Build history of the part. All positions in model axes, mm. Face numbers are marked on the shaded views. Give positions to 0.01 mm unless a question says otherwise; leave off trailing zeros. Loops run counter-clockwise (first coordinate to the right, second up) from the corner with the lowest first, then second, coordinate; pieces in that order, holes last. Notation, with made-up numbers: (-31, 74) -> (-9, 74) arc R19 ccw to (-9, 86) -> close; hole circle Ø7 at (60.25, -19). An arc over 180 degrees is marked (long way). Answer as a JSON object with one key per item and string values. Group by question number.
Q1. Drop flat-ended pins along their axis: pin 1 (2.5 mm diameter, centred on x = 49.5, z = 15, fed in from -Y); pin 2 (1.2 mm diameter, centred on x = 98, z = 32.5, fed in from -Y); pin 3 (2 mm diameter, centred on y = -8.5, z = 10, fed in from -X); pin 4 (2 mm diameter, centred on y = -9, z = 36, fed in from -X). Give the stop position or say it passes through.
Q2. Band-saw the part on D-D, the plane x = 80. Write the cut outline in (y, z).
Q3. Band-saw the part on A-A, the plane x = 49.5. Write the cut outline in (y, z), plus the area to 3 significant figures.
Q4. Two-plate mould, pull along X, no slides. Class the marked faces 1 and 2: pulls with the +X half, pulls with the -X half, needs draft (parallel to the pull), parting line crosses it, or undercut.
Q5. Wall check: probe 1 along Z at (x, y) = (5.5, -4); probe 2 along X at (y, z) = (-4.75, 49); probe 3 along X at (y, z) = (-4.5, 15). Give the ranges that are in metal, low to high. Write a range as from..to.
Q6. Band-saw the part on C-C, the plane x = 18. Write the cut outline in (y, z), plus the area to 3 significant figures.
from build123d import *

# Parameters (mm, degrees)
BOSS_EXTRUDE1_DEPTH                  = 60
FILLET1_R                            = 1
F_2_6_START                          = -7
F_2_6_2_6_DIAMETER_HOLE1_OUTLINE_R   = 1.3
F_2_6_2_6_DIAMETER_HOLE1_DEPTH       = 7
F_2_6_START_2                        = -8.6
F_2_6_2_6_DIAMETER_HOLE1_2_OUTLINE_R = 1.3
F_2_6_2_6_DIAMETER_HOLE1_2_DEPTH     = 1.6


# Read off the part's stored shape, not the designer's step: Ø2.6 (2.6) Diameter Hole1
with BuildPart() as part:
    # Sketch1 → Boss-Extrude1 (new body)
    with BuildSketch(Plane.XY):
        with BuildLine():
            Line((0, 0), (7.751531367, 0))
            Line((7.751531367, 0), (7.751531367, -1.25))
            ThreePointArc((7.751531367, -1.25), (15.339084008, -11.30616411), (26.74540449, -5.958898944))
            Line((26.74540449, -5.958898944), (28.74540449, -5.958898944))
            ThreePointArc((28.74540449, -5.958898944), (39.981472468, -11.346794345), (47.74540449, -1.6))
            Line((47.74540449, -1.6), (51.25459551, -1.6))
            ThreePointArc((51.25459551, -1.6), (59.018527532, -11.346794345), (70.25459551, -5.958898944))
            Line((70.25459551, -5.958898944), (72.25459551, -5.958898944))
            ThreePointArc((72.25459551, -5.958898944), (83.660915992, -11.30616411), (91.248468633, -1.25))
            Line((91.248468633, -1.25), (91.248468633, 0))
            Line((91.248468633, 0), (99, 0))
            Line((99, 0), (99, -1.6))
            Line((99, -1.6), (95.52, -1.6))
            Line((95.52, -1.6), (95.52, -7))
            Line((95.52, -7), (91.970938169, -7))
            ThreePointArc((91.970938169, -7), (83.148029778, -13.449679602), (72.75459551, -10.070537173))
            Line((72.75459551, -10.070537173), (69.75459551, -10.070537173))
            ThreePointArc((69.75459551, -10.070537173), (60.290622518, -13.561218837), (51.507801165, -8.6))
            Line((51.507801165, -8.6), (47.492198835, -8.6))
            ThreePointArc((47.492198835, -8.6), (38.709377482, -13.561218837), (29.24540449, -10.070537173))
            Line((29.24540449, -10.070537173), (26.24540449, -10.070537173))
            ThreePointArc((26.24540449, -10.070537173), (15.851970222, -13.449679602), (7.029061831, -7))
            Line((7.029061831, -7), (3.48, -7))
            Line((3.48, -7), (3.48, -1.6))
            Line((3.48, -1.6), (0, -1.6))
            Line((0, -1.6), (0, 0))
        make_face()
    extrude(amount=BOSS_EXTRUDE1_DEPTH)

    # Fillet1
    fillet1_edges = [part.edges().sort_by_distance(p)[0] for p in [
        (95.52, -1.6, 30),
        (91.970938169, -7, 30),
        (7.029061831, -7, 30),
        (3.48, -1.6, 30),
    ]]
    fillet(fillet1_edges, radius=FILLET1_R)

    # Ø2.6 (2.6) Diameter Hole1 outline → Ø2.6 (2.6) Diameter Hole1 (cut)
    with BuildSketch(Plane(origin=(0, 0, 0), x_dir=(1, 0, 0), z_dir=(0, 1, 0)).offset(F_2_6_START)):
        with Locations((93.5, -15)):
            Circle(F_2_6_2_6_DIAMETER_HOLE1_OUTLINE_R)
        with Locations((93.5, -45)):
            Circle(F_2_6_2_6_DIAMETER_HOLE1_OUTLINE_R)
        with Locations((49.5, -15)):
            Circle(F_2_6_2_6_DIAMETER_HOLE1_OUTLINE_R)
        with Locations((49.5, -45)):
            Circle(F_2_6_2_6_DIAMETER_HOLE1_OUTLINE_R)
    f_2_6_2_6_diameter_hole1 = extrude(amount=F_2_6_2_6_DIAMETER_HOLE1_DEPTH, mode=Mode.SUBTRACT)

    # 2.6 _2.6_ Diameter Hole1 2 outline → 2.6 _2.6_ Diameter Hole1 2 (cut)
    with BuildSketch(Plane(origin=(0, 0, 0), x_dir=(1, 0, 0), z_dir=(0, 1, 0)).offset(F_2_6_START_2)):
        with Locations((49.5, -15)):
            Circle(F_2_6_2_6_DIAMETER_HOLE1_2_OUTLINE_R)
        with Locations((49.5, -45)):
            Circle(F_2_6_2_6_DIAMETER_HOLE1_2_OUTLINE_R)
    f_2_6_2_6_diameter_hole1_2 = extrude(amount=F_2_6_2_6_DIAMETER_HOLE1_2_DEPTH, mode=Mode.SUBTRACT)

    # Mirror1: Ø2.6 (2.6) Diameter Hole1, 2.6 _2.6_ Diameter Hole1 2 across plane
    add(f_2_6_2_6_diameter_hole1.mirror(Plane.ZY.offset(-49.5)), mode=Mode.SUBTRACT)
    add(f_2_6_2_6_diameter_hole1_2.mirror(Plane.ZY.offset(-49.5)), mode=Mode.SUBTRACT)


solid = part.part
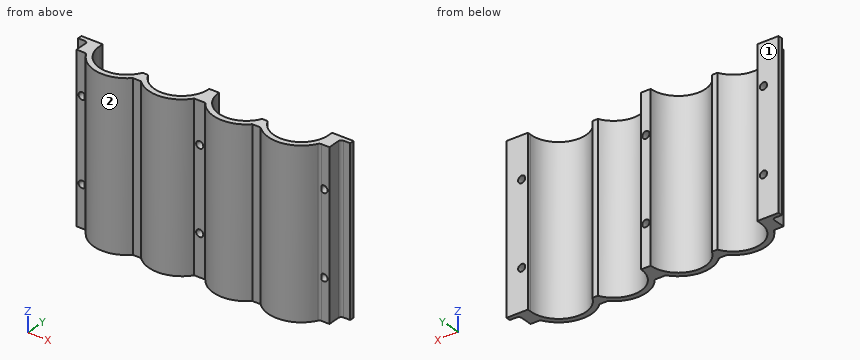
Worked answers:
{
 "1": {"pin 1": "through", "pin 2": "y = -1.6", "pin 3": "x = 7.3", "pin 4": "x = 7.59"},
 "2": {"outline": "(-13.53, 0) -> (-11.52, 0) -> (-11.52, 60) -> (-13.53, 60) -> close"},
 "3": {"outline": "(-8.6, 0) -> (-1.6, 0) -> (-1.6, 13.7) -> (-8.6, 13.7) -> close; (-8.6, 16.3) -> (-1.6, 16.3) -> (-1.6, 43.7) -> (-8.6, 43.7) -> close; (-8.6, 46.3) -> (-1.6, 46.3) -> (-1.6, 60) -> (-8.6, 60) -> close", "area": "384 mm2"},
 "4": {"face 1": "needs draft", "face 2": "undercut"},
 "5": {"probe 1": "0..13.7, 16.3..43.7, 46.3..60", "probe 2": "3.48..8.25, 47.24..51.76, 90.75..95.52", "probe 3": "3.48..4.2, 6.8..8.18, 47.32..48.2, 50.8..51.68, 90.82..92.2, 94.8..95.52"},
 "6": {"outline": "(-13.6, 0) -> (-11.6, 0) -> (-11.6, 60) -> (-13.6, 60) -> close", "area": "120 mm2"}
}
